Could you check a few things on this drawing? It's one solid part, dimensions in mm from its lowest x, y, z. A direction names the side the tool comes from. Give positions to 0.01 mm unless a question says otherwise; leave off trailing zeros. Order: outer loops, then holes, each group sorted by start corner. A loop starts at its lowest first (then second) coordinate and runs counter-clockwise, first axis right, second up.
(1) Imagine slicing it at D-D, the plane z = 0.95. Write out the boundary of the cut face in (x, y), then the cut area to 3 significant figures.
(2) Will these pins go through, and if not, where does the flat tip stop? pin 1 (3.5 mm diameter, centred on x = 5.7, y = 5.7, fed in from +Z); pin 2 (1.5 mm diameter, centred on y = 14.5, z = 2, fed in from -X); pin 3 (1 mm diameter, centred on y = 16, z = 2, fed in from +X).
(3) Imagine slicing it at A-A, the plane y = 11. Write out the boundary of the cut face in (x, z).
(4) If we mould it in two halves opening along Y, with no side actions, what happens to the marked faces 1, 2, 3 and 4? For each: released by +Y, released by -Y, zero draft, split by the parting line, or undercut.
(5) If I drill on probe 1 along X at (y, z) = (5.25, 0.25) (1 decimal); probe 2 along Z at (x, y) = (16.25, 14.5); probe 3 along X at (y, z) = (10, 1.25) (1 decimal), over which ranges is the centre line in solid material (lowest first)?
(6) On a 3-axis mill with a long thin cutter (end or side, diameter ignored), from which of +Z, -Z, +X, -X, +Y, -Y can I reach the whole of each face in a straight line? I mean the marked faces 5 and 6. Say none if no direction works.
(7) Imagine slicing it at C-C, the plane y = 16.5. Write out the boundary of the cut face in (x, z).
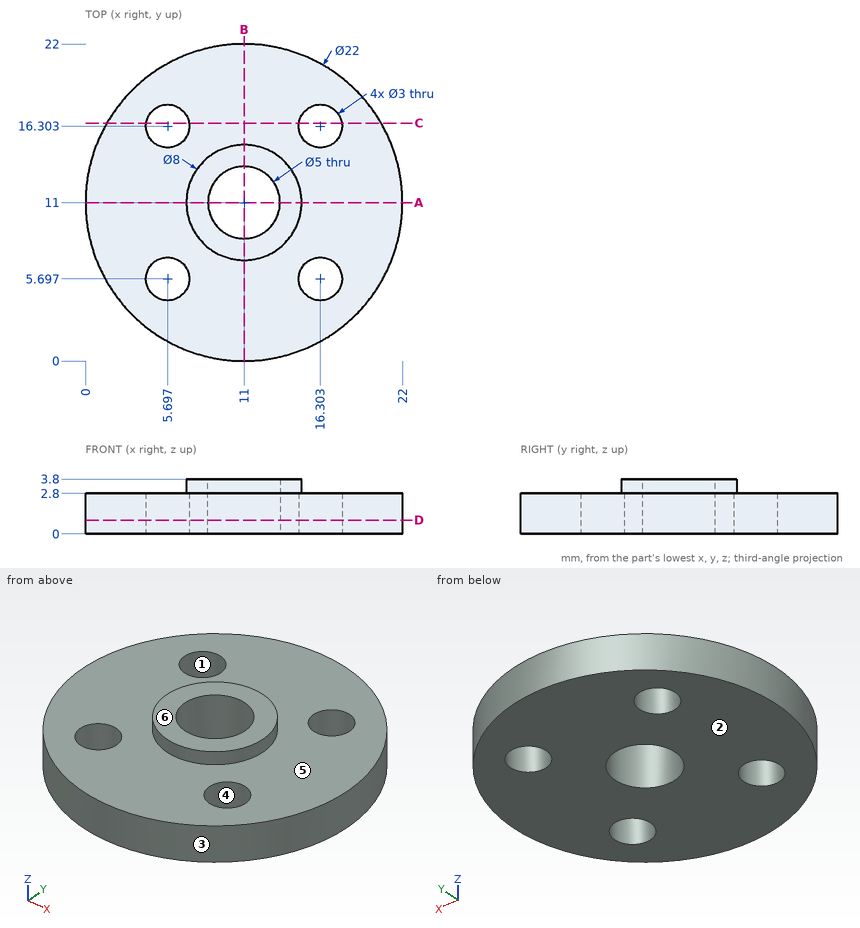
Answer block:
1. outline: circle Ø22 at (11, 11); hole circle Ø3 at (5.7, 5.7); hole circle Ø3 at (5.7, 16.3); hole circle Ø5 at (11, 11); hole circle Ø3 at (16.3, 5.7); hole circle Ø3 at (16.3, 16.3)
1. area: 332 mm2
2. pin 1: stops at z = 2.8
2. pin 2: stops at x = 0.35
2. pin 3: stops at x = 21.04
3. outline: (0, 0) - (8.5, 0) - (8.5, 3.8) - (7, 3.8) - (7, 2.8) - (0, 2.8) - close; (13.5, 0) - (22, 0) - (22, 2.8) - (15, 2.8) - (15, 3.8) - (13.5, 3.8) - close
4. face 1: undercut
4. face 2: zero draft
4. face 3: split by the parting line
4. face 4: undercut
5. probe 1: x = 1.6 to 4.3, 7.1 to 14.9, 17.7 to 20.4
5. probe 2: z = 0 to 2.8
5. probe 3: x = 0 to 8.7, 13.3 to 22
6. face 5: +Z
6. face 6: +Z, +X, -X, +Y, -Y
7. outline: (1.47, 0) - (4.21, 0) - (4.21, 2.8) - (1.47, 2.8) - close; (7.18, 0) - (14.82, 0) - (14.82, 2.8) - (7.18, 2.8) - close; (17.79, 0) - (20.53, 0) - (20.53, 2.8) - (17.79, 2.8) - close
